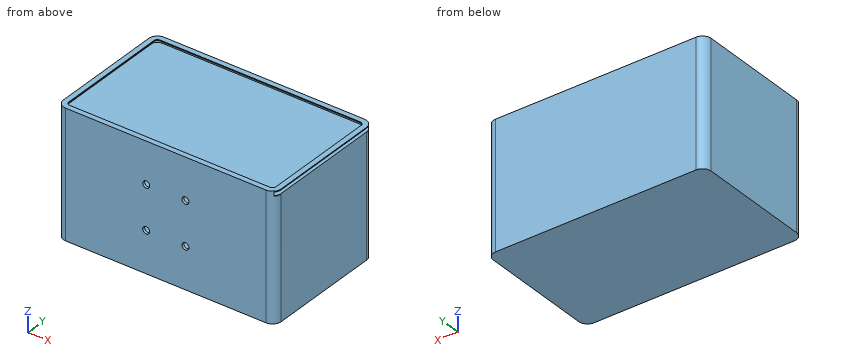
from build123d import *

# Parameters (mm, degrees)
BOSS_EXTRUDE1_DEPTH = 150
SHELL2_T            = -3
BOSS_EXTRUDE2_DEPTH = 3
CUT_EXTRUDE1_DEPTH  = 5
BOSS_EXTRUDE3_DEPTH = 5
BOSS_EXTRUDE4_DEPTH = 1
SKETCH10_W          = 5
SKETCH10_H          = 144
CUT_EXTRUDE2_DEPTH  = 8
SKETCH11_W          = 5
SKETCH11_H          = 144
CUT_EXTRUDE3_DEPTH  = 8
SKETCH12_W          = 1
SKETCH12_H          = 144
BOSS_EXTRUDE5_DEPTH = 16
CUT_EXTRUDE4_DEPTH  = 8
CUT_EXTRUDE5_DEPTH  = 8
SKETCH15_R          = 4
CUT_EXTRUDE13_DEPTH = 9


with BuildPart() as part:
    # Sketch2 → Boss-Extrude1 (new body)
    with BuildSketch(Plane.XY):
        with BuildLine():
            Line((10, 0), (240, 0))
            ThreePointArc((240, 0), (247.071067812, 2.928932188), (250, 10))
            Line((250, 10), (250, 140))
            ThreePointArc((250, 140), (247.071067812, 147.071067812), (240, 150))
            Line((240, 150), (10, 150))
            ThreePointArc((10, 150), (2.928932188, 147.071067812), (0, 140))
            Line((0, 140), (0, 10))
            ThreePointArc((0, 10), (2.928932188, 2.928932188), (10, 0))
        make_face()
    extrude(amount=BOSS_EXTRUDE1_DEPTH)

    # Shell2
    shell2_openings = [part.faces().sort_by_distance(p)[0] for p in [
        (125, 75, 0),
    ]]
    offset(amount=SHELL2_T, openings=shell2_openings, kind=Kind.INTERSECTION)

    # Sketch4 → Boss-Extrude2 (add)
    with BuildSketch(Plane(origin=(0, 0, 0), x_dir=(-1, 0, 0), z_dir=(0, 0, -1))):
        with BuildLine():
            Line((-10, 3), (-240, 3))
            ThreePointArc((-240, 3), (-244.949747468, 5.050252532), (-247, 10))
            Line((-247, 10), (-247, 140))
            ThreePointArc((-247, 140), (-244.949747468, 144.949747468), (-240, 147))
            Line((-240, 147), (-10, 147))
            ThreePointArc((-10, 147), (-5.050252532, 144.949747468), (-3, 140))
            Line((-3, 140), (-3, 10))
            ThreePointArc((-3, 10), (-5.050252532, 5.050252532), (-10, 3))
        make_face()
    extrude(amount=-BOSS_EXTRUDE2_DEPTH)

    # Sketch5 → Cut-Extrude1 (cut)
    with BuildSketch(Plane.XY.offset(150)):
        with BuildLine():
            Line((240, 150), (10, 150))
            ThreePointArc((10, 150), (2.928932188, 147.071067812), (0, 140))
            Line((0, 140), (0, 10))
            ThreePointArc((0, 10), (2.928932188, 2.928932188), (10, 0))
            Line((10, 0), (240, 0))
            ThreePointArc((240, 0), (247.071067812, 2.928932188), (250, 10))
            Line((250, 10), (250, 140))
            ThreePointArc((250, 140), (247.071067812, 147.071067812), (240, 150))
        make_face()
    extrude(amount=-CUT_EXTRUDE1_DEPTH, mode=Mode.SUBTRACT)

    # Sketch6 → Boss-Extrude3 (add)
    with BuildSketch(Plane.XY.offset(135)):
        with BuildLine():
            Line((10, 3), (240, 3))
            ThreePointArc((240, 3), (244.949747468, 5.050252532), (247, 10))
            Line((247, 10), (247, 140))
            ThreePointArc((247, 140), (244.949747468, 144.949747468), (240, 147))
            Line((240, 147), (10, 147))
            ThreePointArc((10, 147), (5.050252532, 144.949747468), (3, 140))
            Line((3, 140), (3, 10))
            ThreePointArc((3, 10), (5.050252532, 5.050252532), (10, 3))
        make_face()
    extrude(amount=BOSS_EXTRUDE3_DEPTH)

    # Sketch7 → Boss-Extrude4 (add)
    with BuildSketch(Plane.XY.offset(144)):
        with BuildLine():
            Line((10, 3), (240, 3))
            ThreePointArc((240, 3), (244.949747468, 5.050252532), (247, 10))
            Line((247, 10), (247, 140))
            ThreePointArc((247, 140), (244.949747468, 144.949747468), (240, 147))
            Line((240, 147), (10, 147))
            ThreePointArc((10, 147), (5.050252532, 144.949747468), (3, 140))
            Line((3, 140), (3, 10))
            ThreePointArc((3, 10), (5.050252532, 5.050252532), (10, 3))
        make_face()
        with BuildLine():
            Line((6, 140), (6, 10))
            ThreePointArc((6, 10), (7.171572875, 7.171572875), (10, 6))
            Line((10, 6), (240, 6))
            ThreePointArc((240, 6), (242.828427125, 7.171572875), (244, 10))
            Line((244, 10), (244, 140))
            ThreePointArc((244, 140), (242.828427125, 142.828427125), (240, 144))
            Line((240, 144), (10, 144))
            ThreePointArc((10, 144), (7.171572875, 142.828427125), (6, 140))
        make_face(mode=Mode.SUBTRACT)
    extrude(amount=BOSS_EXTRUDE4_DEPTH)

    # Sketch10 → Cut-Extrude2 (cut)
    with BuildSketch(Plane(origin=(250, 0, 0), x_dir=(0, 0, -1), z_dir=(1, 0, 0))):
        with Locations((-141.5, 75)):
            Rectangle(SKETCH10_W, SKETCH10_H)
    extrude(amount=-CUT_EXTRUDE2_DEPTH, mode=Mode.SUBTRACT)

    # Sketch11 → Cut-Extrude3 (cut)
    with BuildSketch(Plane(origin=(242, 0, 0), x_dir=(0, 0, -1), z_dir=(1, 0, 0))):
        with Locations((-141.5, 75)):
            Rectangle(SKETCH11_W, SKETCH11_H)
    extrude(amount=-CUT_EXTRUDE3_DEPTH, mode=Mode.SUBTRACT)

    # Sketch12 → Boss-Extrude5 (add)
    with BuildSketch(Plane(origin=(234, 0, 0), x_dir=(0, 0, -1), z_dir=(1, 0, 0))):
        with Locations((-139.5, 75)):
            Rectangle(SKETCH12_W, SKETCH12_H)
    extrude(amount=BOSS_EXTRUDE5_DEPTH)

    # Sketch13 → Cut-Extrude4 (cut)
    with BuildSketch(Plane(origin=(0, 0, 139), x_dir=(-1, 0, 0), z_dir=(0, 0, -1))):
        with BuildLine():
            Line((-250, 3), (-247.141428429, 3))
            ThreePointArc((-247.141428429, 3), (-249.257815193, 6.219410382), (-250, 10))
            Line((-250, 10), (-250, 3))
        make_face()
    extrude(amount=-CUT_EXTRUDE4_DEPTH, mode=Mode.SUBTRACT)

    # Sketch14 → Cut-Extrude5 (cut)
    with BuildSketch(Plane(origin=(0, 0, 139), x_dir=(-1, 0, 0), z_dir=(0, 0, -1))):
        with BuildLine():
            Line((-250, 147), (-250, 140))
            ThreePointArc((-250, 140), (-249.257815193, 143.780589618), (-247.141428429, 147))
            Line((-247.141428429, 147), (-250, 147))
        make_face()
    extrude(amount=-CUT_EXTRUDE5_DEPTH, mode=Mode.SUBTRACT)

    # Sketch15 → Cut-Extrude13 (cut)
    with BuildSketch(Plane.XZ):
        with Locations((102.5, 97.5)):
            Circle(SKETCH15_R)
        with Locations((102.5, 47.5)):
            Circle(SKETCH15_R)
        with Locations((147.5, 47.5)):
            Circle(SKETCH15_R)
        with Locations((147.5, 97.5)):
            Circle(SKETCH15_R)
    extrude(amount=-CUT_EXTRUDE13_DEPTH, mode=Mode.SUBTRACT)


solid = part.part
For this review, take the finished solid that the model builds, in its own axes (mm). Round coordinates to 2 decimals unless told otherwise and drop trailing zeros. Order: outer loops, then holes, each group sorted by start corner. A loop starts at its lowest first (then second) coordinate and runs counter-clockwise, first axis right, second up. Notation, with made-up numbers: (23, -19) -> (75, -19) arc R15 ccw to (75, -9) -> close; hole circle Ø4 at (69.25, 25). An arc over 180 degrees is marked (long way). Put each result on its own line as item: value.
Q1. Add section D-D on z = 47.5. Write out the cut boundary in (x, y).
Check result:
outline: (0, 10) arc R10 ccw to (10, 0) -> (98.5, 0) -> (98.5, 3) -> (10, 3) arc R7 cw to (3, 10) -> (3, 140) arc R7 cw to (10, 147) -> (240, 147) arc R7 cw to (247, 140) -> (247, 10) arc R7 cw to (240, 3) -> (151.5, 3) -> (151.5, 0) -> (240, 0) arc R10 ccw to (250, 10) -> (250, 140) arc R10 ccw to (240, 150) -> (10, 150) arc R10 ccw to (0, 140) -> close; (106.5, 0) -> (143.5, 0) -> (143.5, 3) -> (106.5, 3) -> close
Q2. Add section A-A on x = 102.5. Write out the cut boundary in (y, z), plus the area to 3 significant figures.
Check result:
outline: (0, 0) -> (150, 0) -> (150, 145) -> (144, 145) -> (144, 144) -> (147, 144) -> (147, 140) -> (3, 140) -> (3, 144) -> (6, 144) -> (6, 145) -> (0, 145) -> (0, 101.5) -> (3, 101.5) -> (3, 135) -> (147, 135) -> (147, 3) -> (3, 3) -> (3, 43.5) -> (0, 43.5) -> close; (0, 51.5) -> (3, 51.5) -> (3, 93.5) -> (0, 93.5) -> close
area: 1,980 mm2
Q3. Add section B-B on y = 107. Write out the cut boundary in (x, z), plus the area to 3 significant figures.
Check result:
outline: (0, 0) -> (250, 0) -> (250, 140) -> (3, 140) -> (3, 144) -> (6, 144) -> (6, 145) -> (0, 145) -> close; (244, 144) -> (250, 144) -> (250, 145) -> (244, 145) -> close; hole (3, 3) -> (247, 3) -> (247, 135) -> (3, 135) -> close
area: 2,820 mm2
Q4. Insertion check: pin 1 Ø5 at (x, y) = (174.5, 37.5) entering from +Z; pin 2 Ø6.5 at (x, z) = (102.5, 97.5) entering from -Y. Each pin has a flat end and moves straight along its axis. Give the tip position at first contact, or say it passes through.
Check result:
pin 1: z = 140
pin 2: y = 147
Q5. For probe 1 along Z at (x, y) = (102, 2); probe 2 along Z at (x, y) = (131.5, 57); probe 3 along Y at (x, z) = (43, 47.5), list the stretches that pass through material, from the lowest coordinate up. Write a range as [from, to].
Check result:
probe 1: [0, 43.53], [51.47, 93.53], [101.47, 145]
probe 2: [0, 3], [135, 140]
probe 3: [0, 3], [147, 150]
Q6. Add section C-C on x = 179.5. Write out the cut boundary in (y, z).
Check result:
outline: (0, 0) -> (150, 0) -> (150, 145) -> (144, 145) -> (144, 144) -> (147, 144) -> (147, 140) -> (3, 140) -> (3, 144) -> (6, 144) -> (6, 145) -> (0, 145) -> close; hole (3, 3) -> (147, 3) -> (147, 135) -> (3, 135) -> close
